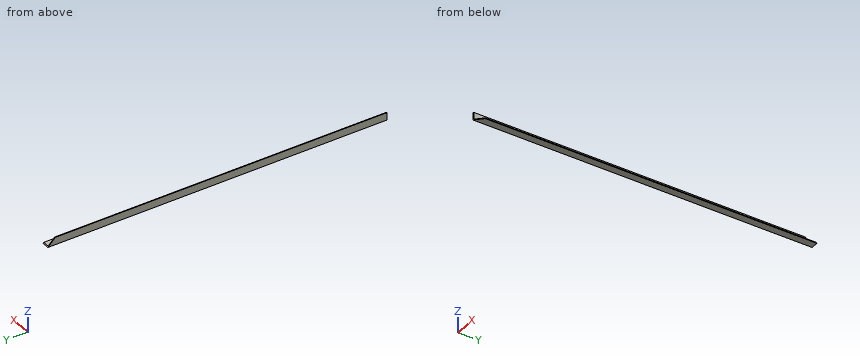
from build123d import *

# Parameters (mm, degrees)
F1_DEPTH = 1380
F2_SIZE  = 29.99999
F3_SIZE  = 29.99999


# Not quite as in the source:
# - a fillet or chamfer is up to 0.001 mm smaller than in the source, because OpenCascade refuses the exact size


with BuildPart() as f1:
    # F0 (on Front) → F1 (new body)
    with BuildSketch(Plane.XZ):
        Polygon((-30, 0), (0, 0), (0, 3), (-27, 3), (-27, 30), (-30, 30), align=None)
    extrude(amount=-F1_DEPTH)

    # F2 (size 30 in the source; OpenCascade refuses exactly that, so slightly less here)
    f2_edges = [f1.edges().sort_by_distance(p)[0] for p in [
        (0, 0, 1.5),
    ]]
    chamfer(f2_edges, length=F2_SIZE)

    # F3 (size 30 in the source; OpenCascade refuses exactly that, so slightly less here)
    f3_edges = [f1.edges().sort_by_distance(p)[0] for p in [
        (-28.5, 1380, 30),
    ]]
    chamfer(f3_edges, length=F3_SIZE)


solid = f1.part
Here's how the part is built. I have some questions about the finished solid (model axes, mm). Give positions to 0.01 mm unless a question says otherwise; leave off trailing zeros. Order: outer loops, then holes, each group sorted by start corner. A loop starts at its lowest first (then second) coordinate and runs counter-clockwise, first axis right, second up. Notation, with made-up numbers: (55.5, 84.5) -> (61.5, 84.5) arc R6 cw to (61.5, 92.5) -> close; hole circle Ø6 at (30.25, -17.75). An arc over 180 degrees is marked (long way). One line per item, written item: value. Start each with the question number.
1. Will these pins go through, and if not, where does the flat tip stop? pin 1 Ø1.5 at (y, z) = (188, 18) entering from +X; pin 2 Ø1 at (x, y) = (-18, 775.5) entering from +Z; pin 3 Ø5 at (x, z) = (-11, 3) entering from +Y.
2. I need wall thicknesses on probe 1 along X at (y, z) = (558, 18.5); probe 2 along Z at (x, y) = (-13, 932); probe 3 along Y at (x, z) = (-20, 2.5). Which ranges of each line are inside material? Lowest first, please. Write a range as from..to.
3. Imagine slicing it at C-C, the plane y = 499. List the corners of the cut face in (x, z) for me.
Values follow:
1. pin 1: stops at x = -27
1. pin 2: stops at z = 3
1. pin 3: stops at y = 1379.5
2. probe 1: x = -30..-27
2. probe 2: z = 0..3
2. probe 3: y = 10..1377.5
3. outline: (-30, 0) -> (0, 0) -> (0, 3) -> (-27, 3) -> (-27, 30) -> (-30, 30) -> close
